Build history of the part. All positions in model axes, mm. A direction names the side the tool comes from. Round coordinates to 2 decimals unless told otherwise and drop trailing zeros. Write each loop counter-clockwise with the first axis right and the second up, starting at its lowest first coordinate (ties: lowest second). Pieces come first, ordered by that corner, then holes. Notation, with made-up numbers: (-40, 10) - (-21, 10) arc R17 ccw to (-21, 42) - close; hole circle Ø7 at (89, 49). An arc over 180 degrees is marked (long way). Answer as a JSON object with one key per item and string values. Group by question number.
Item 1: Which spindle directions (+Z, -Z, +X, -X, +Y, -Y) get a long thin tool onto all of the face, cutting with end or side? Do faces 1 (the flat face through (-27.455, 35.907, 99.3)), 2 (the flat face through (43, 12.576, -3)), 3 (the cylindrical face through (59.075, -7.649, 187.675)), 4 (the flat face through (15.486, -47.339, 99.3)), 5 (the flat face through (42.051, 19.063, 99.3)). Say none if no direction does.
Item 2: Slice it at B-B, the plane z = 91. List the corners of the cut face in (x, y), then the cut area to 3 significant figures.
Item 3: Slice it at C-C, the plane y = 49.5. List the corners of the cut face in (x, z).
Item 4: Flat gauge pins, fed straight in: pin 1 (9.5 mm diameter, centred on y = -45.5, z = -2.5, fed in from -X); pin 2 (6.5 mm diameter, centred on x = 50.5, y = 22, fed in from +Z); pin 3 (10 mm diameter, centred on x = 39, y = 49, fed in from +Z); pin 4 (23 mm diameter, centred on x = -43, y = -14, fed in from +Z). Where does each tip first touch, or does it go through?
Item 5: Slice it at A-A, the plane z = 38. List the corners of the cut face in (x, y).
Item 6: Two-plate mould, pull along Z, no slides. Class faces 6 (the flat face through (-36, 22, 150)), 7 (the flat face through (-43.93, 14.95, 99.3)), 8 (the flat face through (46.254, 31.643, -2.953)), 9 (the flat face through (0, -33, 150)): +Z half, -Z half, draft (parallel to the pull), parting line (faces both ways), or undercut.
Item 7: Probe line 1 (Y direction, x = 0, z = 184.5); line 2 (X direction, y = -14, z = 153); line 3 (Z direction, x = -45, y = -22). List the from-to ranges inside material, lowest first. Write a range as from..to.
from build123d import *

# Parameters (mm, degrees)
F1_DEPTH  = 50
F3_DEPTH  = 100
F4_R      = 35.61174
F5_DEPTH  = 150.001
F6_R      = 34.763964
F6_R_2    = 13.459026
F6_R_3    = 29.528725
F6_R_4    = 31.072571
F7_DEPTH  = 50
F9_DEPTH  = 12.5
F10_R     = 7.524559
F11_DEPTH = 25
F12_R     = 18.555178
F12_R_2   = 23.242661
F12_R_3   = 26.64625
F13_DEPTH = 25


with BuildPart() as f1:
    # F0 (on Top) → F1 (new body)
    with BuildSketch(Plane.XY):
        Polygon((57.372367, 33.123951), (-57.372367, 33.123951), (0, -66.247903), align=None)
    extrude(amount=F1_DEPTH)

    # F2 (on face) → F3 (join)
    with BuildSketch(Plane.XY.offset(50)):
        Polygon((35.541334, 31.556312), (11.41747, 45.344661), (-16.331361, 43.901813), (-38.895099, 27.685861), (-49.109919, 1.845256), (-43.732686, -25.415792), (-24.470635, -45.442094), (2.560671, -51.87544), (28.778981, -42.673288), (45.860168, -20.757257), (48.381076, 6.914469), align=None)
    extrude(amount=F3_DEPTH)

    # F4 (on face) → F5 (cut, through all)
    with BuildSketch(Plane.XY.offset(150)):
        Circle(F4_R)
    extrude(amount=-F5_DEPTH, mode=Mode.SUBTRACT)

    # F6 (on face) → F7 (join)
    with BuildSketch(Plane.XY.offset(150)):
        with Locations((0, 40.323675)):
            Circle(F6_R)
        with Locations((0, -44.642087)):
            Circle(F6_R_2)
        with Locations((41.376553, -13.222456)):
            Circle(F6_R_3)
        with Locations((-39.38517, -13.44372)):
            Circle(F6_R_4)
    extrude(amount=F7_DEPTH)

    # F8 (on face) → F9 (join, symmetric)
    with BuildSketch(Plane(origin=(0, 0, 0), x_dir=(1, 0, 0), z_dir=(0, 0, -1))):
        Polygon((-43.621281, -9.306372), (-51.77561, -23.430084), (-40.862988, -35.549779), (-25.964287, -28.91645), (-27.669006, -12.697132), align=None)
        Polygon((-8.124595, 53.485743), (-8.124595, 41.680016), (3.103319, 38.031846), (10.042551, 47.58288), (3.103319, 57.133913), align=None)
        Polygon((49.025573, -12.575652), (34.519002, -12.575652), (30.036225, -26.37222), (41.772287, -34.898969), (53.50835, -26.37222), align=None)
    extrude(amount=F9_DEPTH, both=True)

    # F10 (on face) → F11 (cut)
    with BuildSketch(Plane.XY.offset(200)):
        with Locations((0, -44.642087)):
            Circle(F10_R)
    extrude(amount=-F11_DEPTH, mode=Mode.SUBTRACT)

    # F12 (on face) → F13 (cut)
    with BuildSketch(Plane.XY.offset(200)):
        with Locations((41.376553, -13.222456)):
            Circle(F12_R)
        with Locations((-40.637251, -14.778094)):
            Circle(F12_R_2)
        with Locations((0, 43.16001)):
            Circle(F12_R_3)
    extrude(amount=-F13_DEPTH, mode=Mode.SUBTRACT)


solid = f1.part
Geometry says:
{
 "1": {"face 1": "-X, +Y", "face 2": "-Z, +X, -Y", "face 3": "+Z", "face 4": "+X, -Y", "face 5": "+X, +Y"},
 "2": {"outline": "(-49.11, 1.85) - (-43.73, -25.42) - (-24.47, -45.44) - (2.56, -51.88) - (28.78, -42.67) - (45.86, -20.76) - (48.38, 6.91) - (35.54, 31.56) - (11.42, 45.34) - (-16.33, 43.9) - (-38.9, 27.69) - close; hole circle Ø71.22 at (0, 0)", "area": "3,250 mm^2"},
 "3": {"outline": "(-33.53, 150) - (33.53, 150) - (33.53, 200) - (25.88, 200) - (25.88, 175) - (-25.88, 175) - (-25.88, 200) - (-33.53, 200) - close"},
 "4": {"pin 1": "stops at x = -14.31", "pin 2": "stops at z = 50", "pin 3": "passes through", "pin 4": "stops at z = 175"},
 "5": {"outline": "(-57.37, 33.12) - (-35.22, -5.24) arc R35.61 cw to (-13.08, 33.12) - close; (-22.15, -27.89) - (0, -66.25) - (22.15, -27.89) arc R35.61 cw to start; (13.08, 33.12) arc R35.61 cw to (35.22, -5.24) - (57.37, 33.12) - close"},
 "6": {"face 6": "+Z half", "face 7": "undercut", "face 8": "draft", "face 9": "-Z half"},
 "7": {"line 1": "y = -58.1..-52.17, -37.12..-31.18, 5.56..16.51, 69.81..75.09", "line 2": "x = -70.45..-8.32, 11.86..70.9", "line 3": "z = 150..175"}
}
